from build123d import *

# Parameters (mm, degrees)
SKETCH_1_W               = 60
SKETCH_1_H               = 30
EXTRUDE_1_DEPTH          = 3
SKETCH_2_R               = 1.5
CUT_EXTRUDE_1_DEPTH      = 3
SKETCH_5_W               = 12
SKETCH_5_H               = 12
EXTRUDE_2_DEPTH          = 4
MIRROR_2_COPY_1_SKETCH_R = 1.5
MIRROR_2_COPY_1_DEPTH    = 3
SKETCH_3_W               = 30.992816336
SKETCH_3_H               = 3
CUT_EXTRUDE_2_DEPTH      = 3
FILLET_1_R               = 1
FILLET_1_OF_MIRROR_3_R   = 1
FILLET_2_R               = 2
SKETCH_4_R               = 2.5
CUT_EXTRUDE_3_DEPTH      = 5
CUT_EXTRUDE_3_DEPTH_BACK = 4
FILLET_3_R               = 1


with BuildPart() as part:
    # 草图1 → 凸台-拉伸1 (new body)
    with BuildSketch(Plane(origin=(0, 0, 0), x_dir=(1, 0, 0), z_dir=(0, 1, 0))):
        Rectangle(SKETCH_1_W, SKETCH_1_H)
    extrude(amount=EXTRUDE_1_DEPTH)

    # 草图2 → 切除-拉伸1 (cut)
    with BuildSketch(Plane(origin=(0, 3, 0), x_dir=(1, 0, 0), z_dir=(0, 1, 0))):
        with Locations((-24, -9)):
            Circle(SKETCH_2_R)
    cut_extrude_1 = extrude(amount=-CUT_EXTRUDE_1_DEPTH, mode=Mode.SUBTRACT)

    # 草图5 → 凸台-拉伸2 (add)
    with BuildSketch(Plane(origin=(0, 3, 0), x_dir=(1, 0, 0), z_dir=(0, 1, 0))):
        Rectangle(SKETCH_5_W, SKETCH_5_H)
    extrude(amount=EXTRUDE_2_DEPTH)

    # 镜向1: 切除-拉伸1 across plane
    add(cut_extrude_1.mirror(Plane.XY), mode=Mode.SUBTRACT)

    # 镜向2: 切除-拉伸1 across plane
    add(cut_extrude_1.mirror(Plane(origin=(0, 0, 0), x_dir=(0, 0, 1), z_dir=(1, 0, 0))), mode=Mode.SUBTRACT)

    # 镜向2 copy 1 sketch → 镜向2 copy 1 (cut)
    with BuildSketch(Plane(origin=(0, 3, 0), x_dir=(-1, 0, 0), z_dir=(0, 1, 0))):
        with Locations((-24, -9)):
            Circle(MIRROR_2_COPY_1_SKETCH_R)
    extrude(amount=-MIRROR_2_COPY_1_DEPTH, mode=Mode.SUBTRACT)

    # 草图3 → 切除-拉伸2 (cut)
    with BuildSketch(Plane(origin=(0, 3, 0), x_dir=(1, 0, 0), z_dir=(0, 1, 0))):
        with Locations((0, -9)):
            Rectangle(SKETCH_3_W, SKETCH_3_H)
    cut_extrude_2 = extrude(amount=-CUT_EXTRUDE_2_DEPTH, mode=Mode.SUBTRACT)

    # 圆角1
    fillet_1_edges = [part.edges().sort_by_distance(p)[0] for p in [
        (-15.496408168, 1.5, 10.5),
        (-15.496408168, 1.5, 7.5),
        (15.496408168, 1.5, 7.5),
        (15.496408168, 1.5, 10.5),
    ]]
    fillet(fillet_1_edges, radius=FILLET_1_R)

    # 镜向3: 切除-拉伸2 across plane
    add(cut_extrude_2.mirror(Plane.XY), mode=Mode.SUBTRACT)

    # 圆角1 of 镜向3
    fillet_1_of_mirror_3_edges = [part.edges().sort_by_distance(p)[0] for p in [
        (-15.496408168, 1.5, -10.5),
        (-15.496408168, 1.5, -7.5),
        (15.496408168, 1.5, -7.5),
        (15.496408168, 1.5, -10.5),
    ]]
    fillet(fillet_1_of_mirror_3_edges, radius=FILLET_1_OF_MIRROR_3_R)

    # 圆角2
    fillet_2_edges = [part.edges().sort_by_distance(p)[0] for p in [
        (-30, 1.5, -15),
        (30, 1.5, -15),
        (30, 1.5, 15),
        (-30, 1.5, 15),
    ]]
    fillet(fillet_2_edges, radius=FILLET_2_R)

    # 草图4 → 切除-拉伸3 (cut, two sides)
    with BuildSketch(Plane(origin=(0, 3, 0), x_dir=(1, 0, 0), z_dir=(0, 1, 0))) as cut_extrude_3_sk:
        Circle(SKETCH_4_R)
    extrude(amount=CUT_EXTRUDE_3_DEPTH, mode=Mode.SUBTRACT)
    extrude(cut_extrude_3_sk.sketch, amount=-CUT_EXTRUDE_3_DEPTH_BACK, mode=Mode.SUBTRACT)

    # 圆角3
    fillet_3_edges = [part.edges().sort_by_distance(p)[0] for p in [
        (-6, 3, 0),
        (-6, 5, -6),
        (0, 3, 6),
        (-6, 5, 6),
        (6, 3, 0),
        (6, 5, 6),
        (0, 3, -6),
        (6, 5, -6),
        (-6, 7, 0),
        (0, 7, 6),
        (6, 7, 0),
        (0, 7, -6),
    ]]
    fillet(fillet_3_edges, radius=FILLET_3_R)


solid = part.part
CAD build for the part. Positions are in the model's coordinates, mm. A direction names the side the tool comes from. Coordinates: 2 decimals unless noted, no trailing zeros. Loops run counter-clockwise (first coordinate to the right, second up) from the corner with the lowest first, then second, coordinate; pieces in that order, holes last. Notation, with made-up numbers: (-20.5, -1) - (-10.5, -1) arc R28 ccw to (-10.5, 28) - close; hole circle Ø8 at (80, -38.5). An arc over 180 degrees is marked (long way). Use one line per item in the form item = value. Start each with the question number.
1) Band-saw the part on B-B (x = 0). Give the cut face in (y, z), and give its area (3 significant figures).
2) Flat gauge pins, fed straight in: pin 1 (1 mm diameter, centred on x = 20, z = 8, fed in from -Y); pin 2 (1 mm diameter, centred on y = 5, z = -2, fed in from +X); pin 3 (1.8 mm diameter, centred on x = -24, z = 9, fed in from +Y); pin 4 (2 mm diameter, centred on y = 5.5, z = 1, fed in from -X). Where does each tip first touch, or does it go through?
3) Drill centre lines: L1, parallel to Z at x = 24, y = 1.3; L2, parallel to X at y = 2, z = 9; L3, parallel to Z at x = -1.5, y = 2. Where is each one in solid material? Low to high. Write a range as from..to.
4) Two-plate mould, pull along X, no slides. Class faces 1 (the face through (-29.43, 1.52, -14.4)), 2 (the face through (29.4, 1.52, 14.43)), 3 (the face through (0, 5, -6)), 4 (the face through (0, 2, -7.5)): +X half, -X half, draft (parallel to the pull), parting line (faces both ways), or undercut.
5) Band-saw the part on A-A (x = 24). Give the cut face in (y, z), and give its area (3 significant figures).
6) Band-saw the part on D-D (y = 2.25). State how many separate pieces and enclosed holes the cut face has, and give its area (3 significant figures).
7) Tool access for faces 5 (the face through (0, 2, -10.5)), 6 (the face through (30, 1, 0)), 7 (the face through (0, 1, -15)), 8 (the face through (-6, 5, 0)), 9 (the face through (0, 5, 6)): list every direction of +Z, -Z, +X, -X, +Y, -Y with a clear straight run to the whole face (end or side of a thin tool).
8) Band-saw the part on C-C (y = 4.75). Give the cut face in (x, z).
Check values:
q1.outline = (0, -15) - (3, -15) - (3, -10.5) - (0, -10.5) - close; (0, -7.5) - (3, -7.5) - (3, -7) arc R1 cw to (4, -6) - (6, -6) arc R1 ccw to (7, -5) - (7, -2.5) - (0, -2.5) - close; (0, 2.5) - (7, 2.5) - (7, 5) arc R1 ccw to (6, 6) - (4, 6) arc R1 cw to (3, 7) - (3, 7.5) - (0, 7.5) - close; (0, 10.5) - (3, 10.5) - (3, 15) - (0, 15) - close
q1.area = 85.0 mm2
q2.pin_1 = 0
q2.pin_2 = 6
q2.pin_3 = through
q2.pin_4 = -6
q3.L1 = -15..-10.5, -7.5..7.5, 10.5..15
q3.L2 = -30..-25.5, -22.5..-15.5, 15.5..22.5, 25.5..30
q3.L3 = -15..-10.5, -7.5..-2, 2..7.5, 10.5..15
q4.face_1 = -X half
q4.face_2 = +X half
q4.face_3 = draft
q4.face_4 = undercut
q5.outline = (0, -15) - (3, -15) - (3, -10.5) - (0, -10.5) - close; (0, -7.5) - (3, -7.5) - (3, 7.5) - (0, 7.5) - close; (0, 10.5) - (3, 10.5) - (3, 15) - (0, 15) - close
q5.area = 72.0 mm2
q6.separate_pieces = 1
q6.enclosed_holes = 7
q6.area = 1,560 mm2
q7.face_5 = +Y, -Y
q7.face_6 = +Z, -Z, +X, +Y, -Y
q7.face_7 = -Z, +X, -X, +Y, -Y
q7.face_8 = +Z, -Z, -X, +Y
q7.face_9 = +Z, +X, -X, +Y
q8.outline = (-6, -5) arc R1 ccw to (-5, -6) - (5, -6) arc R1 ccw to (6, -5) - (6, 5) arc R1 ccw to (5, 6) - (-5, 6) arc R1 ccw to (-6, 5) - close; hole circle Ø5 at (0, 0)
